Here's how the part is built. I have some questions about the finished solid (model axes, mm). A direction names the side the tool comes from. Round coordinates to 2 decimals unless told otherwise and drop trailing zeros. Loops run counter-clockwise (first coordinate to the right, second up) from the corner with the lowest first, then second, coordinate; pieces in that order, holes last. Notation, with made-up numbers: (86.25, -19) -> (108.25, -19) arc R22 cw to (108.25, 16) -> close; hole circle Ø4 at (88, -33). An arc over 180 degrees is marked (long way). Use one line per item in the form item = value. Start each with the question number.
Item 1: If we section it at B-B (z = 3): Write out the boundary of the cut face in (x, y).
Item 2: If we section it at C-C (x = 4.5): Write out the boundary of the cut face in (y, z), then the cut area to 3 significant figures.
Item 3: For faces 4 (the face through (6.67, 28.38, 8.33)), 5 (the face through (-6.23, 33.83, 9.1)), 6 (the face through (-3.5, 28, 7)), 7 (the face through (5, 7, 7)), 8 (the face through (-5, 7, 7)), which set-ups out of +Z, -Z, +X, -X, +Y, -Y let a thin tool reach every point of the face, with its end or its side?
Item 4: If we section it at D-D (y = -2): Write out the boundary of the cut face in (x, z).
Item 5: If I drill on L1, parallel to X at y = 6, z = 3; L2, parallel to Z at x = 0.5, y = 12; L3, parallel to Z at x = 1, y = -2, over which ranges is the centre line in solid material (lowest first)? Write a range as [from, to].
Item 6: I'm going to push flat-ended pins straight in: pin 1 Ø4 at (y, z) = (26, 10.5) entering from +X; pin 2 Ø1 at (x, y) = (-4.5, 25) entering from -Z; pin 3 Ø1.8 at (y, z) = (31, 7.5) entering from -X; pin 4 Ø4.5 at (x, z) = (6, 9) entering from -Y. Where does each tip first touch, or does it pass through?
Item 7: If we section it at A-A (y = 5): Write out the boundary of the cut face in (x, z), then the cut area to 3 significant figures.
Item 8: Thinking about a two-plate mould opening in Z: for faces 1 (the face through (0, 23.32, 7)), 2 (the face through (0, -5, 11)), 3 (the face through (4.84, 29.5, 7.57)), which applies, released by +Z, released by -Z, zero draft, split by the parting line, or undercut?
```python
from build123d import *

# Parameters (mm, degrees)
SKETCH1_W           = 6.5
SKETCH1_H           = 14
BOSS_EXTRUDE1_DEPTH = 15
FILLET1_R           = 10
SKETCH2_R           = 2
CUT_EXTRUDE1_DEPTH  = 18.783419244
SKETCH4_R           = 7.5
BOSS_EXTRUDE2_DEPTH = 29
SKETCH6_W           = 7
SKETCH6_H           = 12.68
CUT_EXTRUDE2_DEPTH  = 40.714606885
CUT_EXTRUDE3_DEPTH  = 34.5
SKETCH8_R           = 1.5
CUT_EXTRUDE4_DEPTH  = 21
SKETCH9_R           = 2.75
CUT_EXTRUDE5_DEPTH  = 10
CUT_EXTRUDE6_DEPTH  = 10
SKETCH11_R          = 1.25
CUT_EXTRUDE7_DEPTH  = 40


with BuildPart() as part:
    # Sketch1 → Boss-Extrude1 (new body)
    with BuildSketch(Plane.XY):
        Rectangle(SKETCH1_W, SKETCH1_H)
    extrude(amount=BOSS_EXTRUDE1_DEPTH)

    # Fillet1
    fillet1_edges = [part.edges().sort_by_distance(p)[0] for p in [
        (0, -7, 15),
    ]]
    fillet(fillet1_edges, radius=FILLET1_R)

    # Sketch2 → Cut-Extrude1 (cut, through all)
    with BuildSketch(Plane(origin=(3.25, 0, 0), x_dir=(0, 0, -1), z_dir=(1, 0, 0))):
        with Locations(Location((-7.5, -2, 0), (0, 0, 90))):
            Circle(SKETCH2_R)
    extrude(amount=-CUT_EXTRUDE1_DEPTH, mode=Mode.SUBTRACT)

    # Sketch4 → Boss-Extrude2 (add)
    with BuildSketch(Plane(origin=(0, 7, 0), x_dir=(1, 0, 0), z_dir=(0, 1, 0))):
        with Locations(Location((0, -7.5, 0), (0, 0, 270))):
            Circle(SKETCH4_R)
    extrude(amount=BOSS_EXTRUDE2_DEPTH)

    # Sketch6 → Cut-Extrude2 (cut, through all)
    with BuildSketch(Plane(origin=(0, 0, 0), x_dir=(-1, 0, 0), z_dir=(0, 0, -1))):
        with Locations((0, 29.66)):
            Rectangle(SKETCH6_W, SKETCH6_H)
    extrude(amount=-CUT_EXTRUDE2_DEPTH, mode=Mode.SUBTRACT)

    # Sketch7 → Cut-Extrude3 (cut, through all)
    with BuildSketch(Plane(origin=(0, 7, 0), x_dir=(1, 0, 0), z_dir=(0, 1, 0))):
        with BuildLine():
            ThreePointArc((0, -15), (-1.666673801, -14.812468697), (-3.25, -14.259252917))
            Line((-3.25, -14.259252917), (-3.25, -15))
            Line((-3.25, -15), (0, -15))
        make_face()
        with BuildLine():
            ThreePointArc((3.25, -14.259252917), (1.666673801, -14.812468697), (0, -15))
            Line((0, -15), (3.25, -15))
            Line((3.25, -15), (3.25, -14.259252917))
        make_face()
        with BuildLine():
            ThreePointArc((-3.25, -0.740747083), (-1.666673801, -0.187531303), (0, 0))
            Line((0, 0), (-3.25, 0))
            Line((-3.25, 0), (-3.25, -0.740747083))
        make_face()
        with BuildLine():
            Line((3.25, 0), (0, 0))
            ThreePointArc((0, 0), (1.666673801, -0.187531303), (3.25, -0.740747083))
            Line((3.25, -0.740747083), (3.25, 0))
        make_face()
    extrude(amount=-CUT_EXTRUDE3_DEPTH, mode=Mode.SUBTRACT)

    # Sketch8 → Cut-Extrude4 (cut, symmetric)
    with BuildSketch(Plane(origin=(-3.5, 0, 0), x_dir=(0, 0, -1), z_dir=(1, 0, 0))):
        with Locations(Location((-7.5, 31, 0), (0, 0, 90))):
            Circle(SKETCH8_R)
    extrude(amount=CUT_EXTRUDE4_DEPTH, both=True, mode=Mode.SUBTRACT)

    # Sketch9 → Cut-Extrude5 (cut)
    with BuildSketch(Plane.ZY.offset(-6.15)):
        with Locations(Location((7.5, 31, 0), (0, 0, 270))):
            Circle(SKETCH9_R)
    extrude(amount=-CUT_EXTRUDE5_DEPTH, mode=Mode.SUBTRACT)

    # Sketch10 → Cut-Extrude6 (cut)
    with BuildSketch(Plane(origin=(-5, 0, 0), x_dir=(0, 0, -1), z_dir=(1, 0, 0))):
        Polygon((-7.5, 34.75277675), (-10.75, 32.876388375), (-10.75, 29.123611625), (-7.5, 27.24722325), (-4.25, 29.123611625), (-4.25, 32.876388375), align=None)
    extrude(amount=-CUT_EXTRUDE6_DEPTH, mode=Mode.SUBTRACT)

    # Sketch11 → Cut-Extrude7 (cut)
    with BuildSketch(Plane.XZ.offset(7)):
        with Locations(Location((0, 12.74882624, 0), (0, 0, 270))):
            Circle(SKETCH11_R)
        with Locations(Location((0, 3, 0), (0, 0, 270))):
            Circle(SKETCH11_R)
    extrude(amount=-CUT_EXTRUDE7_DEPTH, mode=Mode.SUBTRACT)


solid = part.part
```
Values found:
q1.outline = (-6, 7) -> (-3.25, 7) -> (-3.25, -7) -> (-1.25, -7) -> (-1.25, 23.32) -> (-3.5, 23.32) -> (-3.5, 36) -> (-6, 36) -> close; (1.25, -7) -> (3.25, -7) -> (3.25, 7) -> (6, 7) -> (6, 36) -> (3.5, 36) -> (3.5, 23.32) -> (1.25, 23.32) -> close
q2.outline = (7, 1.5) -> (36, 1.5) -> (36, 13.5) -> (7, 13.5) -> close; hole circle Ø3 at (31, 7.5)
q2.area = 341 mm2
q3.face_4 = +X
q3.face_5 = -X
q3.face_6 = +Z, -Z, +Y
q3.face_7 = +Z, -Z, +X, -Y
q3.face_8 = +Z, -Z, -X, -Y
q4.outline = (-3.25, 0.74) arc R7.5 ccw to (3.25, 0.74) -> (3.25, 5.5) -> (-3.25, 5.5) -> close; (-3.25, 9.5) -> (3.25, 9.5) -> (3.25, 13.66) -> (0.86, 13.66) arc R1.25 cw (long way) to (-0.86, 13.66) -> (-3.25, 13.66) -> close; hole circle Ø2.5 at (0, 3)
q5.L1 = [-3.25, -1.25], [1.25, 3.25]
q5.L2 = [0.02, 1.85], [4.15, 11.6], [13.89, 14.98]
q5.L3 = [0.07, 2.25], [3.75, 5.5], [9.5, 12], [13.5, 13.66]
q6.pin_1 = 7.43
q6.pin_2 = 1.16
q6.pin_3 = through
q6.pin_4 = 7
q7.outline = (-3.25, 0.74) arc R7.5 ccw to (3.25, 0.74) -> (3.25, 14.26) arc R7.5 ccw to (-3.25, 14.26) -> close; hole circle Ø2.5 at (0, 3); hole circle Ø2.5 at (0, 12.75)
q7.area = 84.5 mm2
q8.face_1 = zero draft
q8.face_2 = released by +Z
q8.face_3 = undercut
